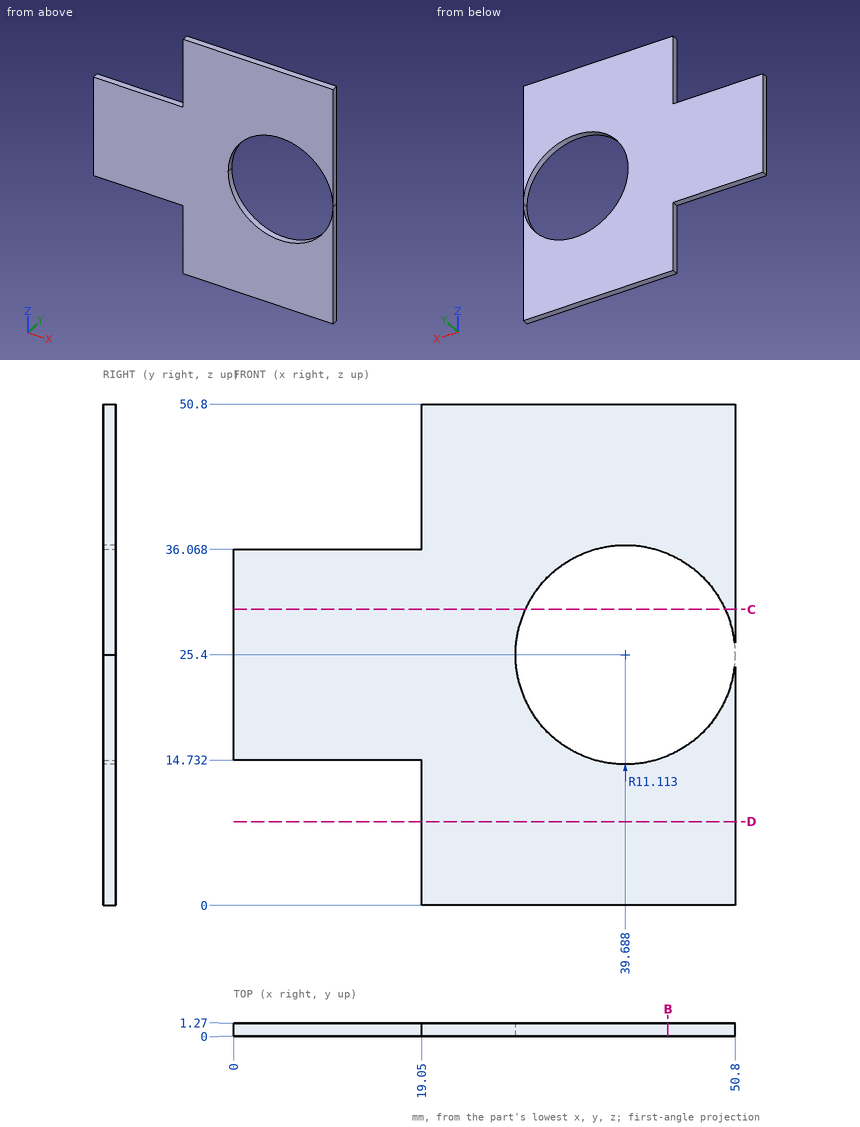
Here's the drawing with two shaded views (mm, measured from the low corner). I have some questions. Give positions to 0.01 mm unless a question says otherwise; leave off trailing zeros. Loops run counter-clockwise (first coordinate to the right, second up) from the corner with the lowest first, then second, coordinate; pieces in that order, holes last. Notation, with made-up numbers: M 28.25,5.5 L 62.25,5.5 A9 cw 62.25,17.5 Z; hole C 86.25,79 d2. An arc over 180 degrees is marked long. Use one line per item in the form item = value. Start each with the question number.
Q1. Will these pins go through, and if not, where does the flat tip stop? pin 1 Ø5 at (x, z) = (12.5, 14) entering from -Y; pin 2 Ø0.6 at (y, z) = (1, 43) entering from -X; pin 3 Ø0.6 at (x, y) = (13.5, 0.5) entering from +Z.
Q2. If we section it at B-B (x = 44): Write out the boundary of the cut face in (y, z).
Q3. I need wall thicknesses on line 1 along X through (y, z) = (1, 2); line 2 along Z through (x, y) = (9, 0.9); line 3 along Z through (x, y) = (39, 0.7). Which ranges of each line are inside material? Lowest first, please.
Q4. If we section it at C-C (z = 30): Write out the boundary of the cut face in (x, y).
Q5. If we section it at D-D (z = 8.5): Write out the boundary of the cut face in (x, y).
Taken from the geometry:
q1.pin_1 = 0
q1.pin_2 = 19.05
q1.pin_3 = 36.07
q2.outline = M 0,0 L 1.27,0 L 1.27,15.16 L 0,15.16 Z; M 0,35.64 L 1.27,35.64 L 1.27,50.8 L 0,50.8 Z
q3.line_1 = 19.05 to 50.8
q3.line_2 = 14.73 to 36.07
q3.line_3 = 0 to 14.31, 36.49 to 50.8
q4.outline = M 0,0 L 29.57,0 L 29.57,1.27 L 0,1.27 Z; M 49.8,0 L 50.8,0 L 50.8,1.27 L 49.8,1.27 Z
q5.outline = M 19.05,0 L 50.8,0 L 50.8,1.27 L 19.05,1.27 Z
